```python
from build123d import *

# Parameters (mm, degrees)
F0_R     = 64.9505041371
F1_DEPTH = 12.7
F3_D     = 38.1
F4_SIZE  = 5.08


with BuildPart() as f1:
    # F0 (on Front) → F1 (new body)
    with BuildSketch(Plane.XZ):
        with Locations((-152.9169678688, -21.0192166269)):
            Circle(F0_R)
    extrude(amount=F1_DEPTH)

    # F3 (through all)
    with Locations(Plane(origin=(0, 0, 0), x_dir=(1, 0, 0), z_dir=(0, 1, 0))):
        with Locations((-151.7456322908, 18.0257931352), (-118.2411909103, -22.082446143), (-189.2130970955, -20.4620826989), (-188.8890266418, 59.5838613808), (-117.2689720988, 56.019064039)):
            Hole(F3_D / 2)

    # F4
    f4_edges = [f1.edges().sort_by_distance(p)[0] for p in [
        (-130.862366, -12.7, -42.672824),
        (-87.985724, -12.7, -19.437569),
        (-130.182417, -12.7, 7.239615),
        (-154.308279, -12.7, 43.916384),
        (-176.668586, -12.7, 6.125495),
        (-217.866858, -12.7, -20.736903),
        (-175.895036, -12.7, -45.653365),
        (-150.069359, -12.7, -85.907267),
        (-170.795632, -12.7, -18.025793),
        (-87.985724, 0, -19.437569),
        (-130.182417, 0, 7.239615),
        (-154.308279, 0, 43.916384),
        (-176.668586, 0, 6.125495),
        (-217.866858, 0, -20.736903),
        (-175.895036, 0, -45.653365),
        (-150.069359, 0, -85.907267),
        (-130.862366, 0, -42.672824),
        (-170.795632, 0, -18.025793),
    ]]
    chamfer(f4_edges, length=F4_SIZE)


solid = f1.part
```
For this review, take the finished solid that the model builds, in its own axes (mm). Round coordinates to 2 decimals unless told otherwise and drop trailing zeros. Write each loop counter-clockwise with the first axis right and the second up, starting at its lowest first coordinate (ties: lowest second). Pieces come first, ordered by that corner, then holes. Notation, with made-up numbers: (25, 88.25) - (58, 88.25) arc R21 cw to (58, 107.25) - close; hole circle Ø6 at (56, 43.25). An arc over 180 degrees is marked (long way). Answer as a JSON object with one key per item and string values.
1. We need section B-B on z = -47. Count the separate pieces of the cut face and the enclosed holes in it, then the cut area to 3 significant figures.
Response values:
{"separate pieces": "3", "enclosed holes": "0", "area": "554 mm2"}
2. We need section A-A on y = -10.5. Give the boundary of the cut face in (x, z) (1 decimal).
Response values:
{"outline": "(-208.2, -49.2) arc R21.9 cw (long way) to (-177.2, -78.1) arc R62.1 ccw to (-125.1, -76.5) arc R21.9 cw (long way) to (-96.9, -47.8) arc R62.1 ccw to (-99.5, 10.6) arc R21.9 cw (long way) to (-133.4, 37.9) arc R62.1 ccw to (-174.9, 37) arc R21.9 cw (long way) to (-207.6, 8.4) arc R62.1 ccw to start; hole circle Ø43.9 at (-151.7, -18)"}
3. We need section C-C on y = -3.5. Give the boundary of the cut face in (x, z).
Response values:
{"outline": "(-208.13, -52.13) arc R20.63 cw (long way) to (-180.12, -78.26) arc R63.37 ccw to (-121.7, -76.17) arc R20.63 cw (long way) to (-97.21, -51.22) arc R63.37 ccw to (-99.6, 13.24) arc R20.63 cw (long way) to (-130.87, 38.39) arc R63.37 ccw to (-177.45, 37.41) arc R20.63 cw (long way) to (-207.57, 11.05) arc R63.37 ccw to start; hole circle Ø41.26 at (-151.75, -18.03)"}
4. For pin 1 Ø6 at (x, y) = (-188, -7) entering from -Z; pin 2 Ø4 at (x, y) = (-168.5, -7) entering from -Z; pin 3 Ø3 at (y, z) = (-6, -13) entering from -X; pin 4 Ø12 at (x, z) = (-167.5, 10) entering from -Y, all flat-tipped, find the tip position at first contact; note any pin that passes through.
Response values:
{"pin 1": "stops at z = -40.94", "pin 2": "stops at z = -84.53", "pin 3": "stops at x = -217.54", "pin 4": "stops at y = -12.7"}
5. Draft analysis for pull direction X (two halves, no side actions). For faces 1 (the face through (-180, 0, -20)), 2 (the face through (-153.874, -10.76, 40.784)), 3 (the face through (-130.79, -7.94, 7.33)), state which applies: +X half, -X half, draft (parallel to the pull), parting line (faces both ways), or undercut.
Response values:
{"face 1": "draft", "face 2": "parting line", "face 3": "undercut"}
6. To check wall thickness, follow line 1 along Z through (x, y) = (-131, -8); line 2 along Z through (x, y) = (-177, -7.5); line 3 along Z through (x, y) = (-167.5, -7.5). State the ranges of each line that lie inside material, in increasing order.
Response values:
{"line 1": "z = -81.76 to -69.77, -42.27 to 7.43, 36.74 to 39.72", "line 2": "z = -81.34 to -74.47, -44.7 to 5.84, 35.08 to 39.3", "line 3": "z = -84.31 to -28.74, -7.32 to 42.27"}
